Check sheet for the modelled part. Datum: model origin and axes. Units: mm. Face numbers are marked on the shaded views. A direction names the side the tool comes from. Give positions to 0.01 mm unless a question says otherwise; leave off trailing zeros. Loops run counter-clockwise (first coordinate to the right, second up) from the corner with the lowest first, then second, coordinate; pieces in that order, holes last. Notation, with made-up numbers: M 38,20 L 60,20 A23 cw 60,58 Z; hole C 23,28.5 d6. An arc over 180 degrees is marked long. Use one line per item in the form item = value.
from build123d import *

# Parameters (mm, degrees)
SKETCH_1_W             = 50
SKETCH_1_H             = 35
EXTRUDE_445_DEPTH      = 11.3
SKETCH_2_R             = 7.5
SKETCH_2_R_2           = 1.25
CUT_EXTRUDE_665_DEPTH  = 36.800698317
CUT_EXTRUDE_1135_DEPTH = 9.3
SKETCH_4_W             = 27
SKETCH_4_H             = 34.5
CUT_EXTRUDE_1595_DEPTH = 1
SKETCH_5_W             = 23
SKETCH_5_H             = 3.5
CUT_EXTRUDE_1822_DEPTH = 12.75
FILLET_1_R             = 1
FILLET_3_R             = 1
SKETCH_7_R             = 1.25
CUT_EXTRUDE_3943_DEPTH = 45.471226653
SKETCH_8_W             = 6
SKETCH_8_H             = 7.8
CUT_EXTRUDE_4259_DEPTH = 3
CHAMFER_1_SIZE         = 1
FILLET_2_R             = 2


with BuildPart() as part:
    # Эскиз1 → Extrude 445 (new body)
    with BuildSketch(Plane.XY):
        with Locations((0, 5.5)):
            Rectangle(SKETCH_1_W, SKETCH_1_H)
    extrude(amount=EXTRUDE_445_DEPTH)

    # Эскиз2 → Cut-Extrude 665 (cut, through all)
    with BuildSketch(Plane(origin=(0, 0, 0), x_dir=(-1, 0, 0), z_dir=(0, 0, -1))):
        Circle(SKETCH_2_R)
        with Locations((-10.5, 6.75)):
            Circle(SKETCH_2_R_2)
        with Locations((10.5, 6.75)):
            Circle(SKETCH_2_R_2)
        with Locations((10.5, -6.75)):
            Circle(SKETCH_2_R_2)
        with Locations((-10.5, -6.75)):
            Circle(SKETCH_2_R_2)
    extrude(amount=-CUT_EXTRUDE_665_DEPTH, mode=Mode.SUBTRACT)

    # Эскиз3 → Cut-Extrude 1135 (cut)
    with BuildSketch(Plane(origin=(0, 0, 0), x_dir=(-1, 0, 0), z_dir=(0, 0, -1))):
        with BuildLine():
            Line((-13.5, 10.25), (13.5, 10.25))
            Line((13.5, 10.25), (13.5, 8.25))
            Line((13.5, 8.25), (10.5, 8.25))
            ThreePointArc((10.5, 8.25), (9, 6.75), (10.5, 5.25))
            Line((10.5, 5.25), (13.5, 5.25))
            Line((13.5, 5.25), (13.5, -5.25))
            Line((13.5, -5.25), (10.5, -5.25))
            ThreePointArc((10.5, -5.25), (9.439339828, -5.689339828), (9, -6.75))
            Line((9, -6.75), (9, -9))
            Line((9, -9), (-9, -9))
            Line((-9, -9), (-9, -6.75))
            ThreePointArc((-9, -6.75), (-9.439339828, -5.689339828), (-10.5, -5.25))
            Line((-10.5, -5.25), (-13.5, -5.25))
            Line((-13.5, -5.25), (-13.5, 5.25))
            Line((-13.5, 5.25), (-10.5, 5.25))
            ThreePointArc((-10.5, 5.25), (-9, 6.75), (-10.5, 8.25))
            Line((-10.5, 8.25), (-13.5, 8.25))
            Line((-13.5, 8.25), (-13.5, 10.25))
        make_face()
    extrude(amount=-CUT_EXTRUDE_1135_DEPTH, mode=Mode.SUBTRACT)

    # Эскиз4 → Cut-Extrude 1595 (cut)
    with BuildSketch(Plane(origin=(0, 0, 0), x_dir=(-1, 0, 0), z_dir=(0, 0, -1))):
        with Locations((0, 5.75)):
            Rectangle(SKETCH_4_W, SKETCH_4_H)
    extrude(amount=-CUT_EXTRUDE_1595_DEPTH, mode=Mode.SUBTRACT)

    # Эскиз5 → Cut-Extrude 1822 (cut)
    with BuildSketch(Plane(origin=(0, 23, 0), x_dir=(1, 0, 0), z_dir=(0, 1, 0))):
        with Locations((0, -1.75)):
            Rectangle(SKETCH_5_W, SKETCH_5_H)
    extrude(amount=-CUT_EXTRUDE_1822_DEPTH, mode=Mode.SUBTRACT)

    # Скругление1
    fillet_1_edges = [part.edges().sort_by_distance(p)[0] for p in [
        (0, 10.25, 3.5),
        (7.5, 0, 9.3),
    ]]
    fillet(fillet_1_edges, radius=FILLET_1_R)

    # Скругление3
    fillet_3_edges = [part.edges().sort_by_distance(p)[0] for p in [
        (13.5, 9.25, 9.3),
        (13.5, 8.25, 5.15),
        (0, 10.25, 9.3),
        (-13.5, 9.25, 9.3),
        (-12, 8.25, 9.3),
        (-13.5, 8.25, 5.15),
        (-9, 6.75, 9.3),
        (-12, 5.25, 9.3),
        (-13.5, 0, 9.3),
        (-13.5, 5.25, 5.15),
        (-12, -5.25, 9.3),
        (-13.5, -5.25, 5.15),
        (-9.439339828, -5.689339828, 9.3),
        (-9, -7.875, 9.3),
        (0, -9, 9.3),
        (-9, -9, 5.15),
        (9, -7.875, 9.3),
        (9, -9, 5.15),
        (9.439339828, -5.689339828, 9.3),
        (12, -5.25, 9.3),
        (13.5, 0, 9.3),
        (13.5, -5.25, 5.15),
        (12, 5.25, 9.3),
        (13.5, 5.25, 5.15),
        (9, 6.75, 9.3),
        (12, 8.25, 9.3),
    ]]
    fillet(fillet_3_edges, radius=FILLET_3_R - 0.0001)  # a hair under: the kernel refuses the full size

    # Эскиз7 → Cut-Extrude 3943 (cut, through all)
    with BuildSketch(Plane(origin=(0, 23, 0), x_dir=(1, 0, 0), z_dir=(0, 1, 0))):
        with Locations(Location((-20, -5.65, 0), (0, 0, 180))):
            Circle(SKETCH_7_R)
        with Locations(Location((20, -5.65, 0), (0, 0, 180))):
            Circle(SKETCH_7_R)
    extrude(amount=-CUT_EXTRUDE_3943_DEPTH, mode=Mode.SUBTRACT)

    # Эскиз8 → Cut-Extrude 4259 (cut)
    with BuildSketch(Plane(origin=(0, 23, 0), x_dir=(1, 0, 0), z_dir=(0, 1, 0))):
        with Locations((0, -7.4)):
            Rectangle(SKETCH_8_W, SKETCH_8_H)
    extrude(amount=-CUT_EXTRUDE_4259_DEPTH, mode=Mode.SUBTRACT)

    # Фаска1
    chamfer_1_edges = [part.edges().sort_by_distance(p)[0] for p in [
        (11.75, 6.75, 11.3),
        (-9.25, 6.75, 11.3),
        (-9.25, -6.75, 11.3),
        (11.75, -6.75, 11.3),
    ]]
    chamfer(chamfer_1_edges, length=CHAMFER_1_SIZE)

    # Скругление2
    fillet_2_edges = [part.edges().sort_by_distance(p)[0] for p in [
        (25, 5.5, 11.3),
        (-25, 5.5, 11.3),
        (25, 5.5, 0),
        (-25, 5.5, 0),
    ]]
    fillet(fillet_2_edges, radius=FILLET_2_R)


solid = part.part
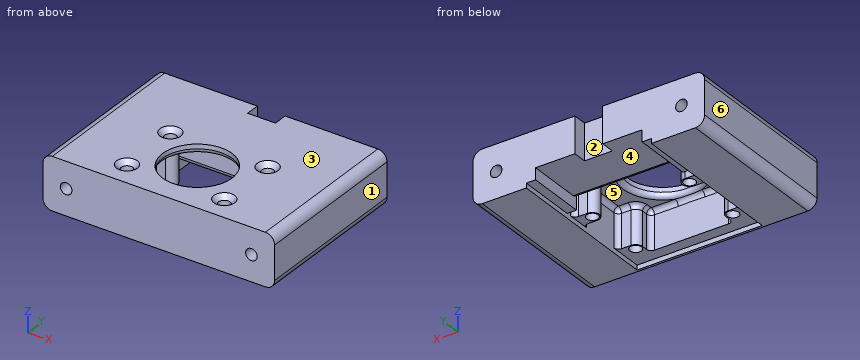
1) Scan lines: line 1 (Y direction, x = 10.5, z = 7.75); line 2 (Y direction, x = 6.5, z = 5.25). Record each from-to range of solid material in increasing order.
Evaluation:
line_1 = -12 to -8, -5.5 to -5.25, 5.25 to 5.5, 8 to 8.25, 10.25 to 23
line_2 = -12 to -9, 10.25 to 23
2) Release check for a two-part mould opening along X. For the marked faces 1, 2 and 3 record: pulls with the +X half, pulls with the -X half, needs draft (parallel to the pull), parting line crosses it, or undercut.
Evaluation:
face_1 = pulls with the +X half
face_2 = undercut
face_3 = needs draft
3) Set-up check for the marked faces 4, 5 and 6: record each of +Z, -Z, +X, -X, +Y, -Y from which the full face is reachable in a straight line by a thin tool's end or side.
Evaluation:
face_4 = -Z, +Y
face_5 = -Z
face_6 = +Z, -Z, -X, +Y, -Y
4) Depth check by flat-ended pin: pin 1 Ø13 at (x, y) = (-3, 16) entering from -Z; pin 2 Ø4 at (x, y) = (-10.5, -6.75) entering from -Z; pin 3 Ø1.5 at (x, y) = (-5.5, -4.5) entering from -Z. Enter the tip coordinate at first touch or a pass-through.
Evaluation:
pin_1 = 3.5
pin_2 = 1
pin_3 = 9.53
5) Section check B-B (x = -20). Record the cut outline in (y, z), then the cut area to 3 significant figures.
Evaluation:
outline = M -12,0 L 23,0 L 23,4.4 L -12,4.4 Z; M -12,6.9 L 23,6.9 L 23,11.3 L -12,11.3 Z
area = 308 mm^2
6) Section check D-D (y = 0). Record the cut outline in (x, z), then the cut area to 3 significant figures.
Evaluation:
outline = M -25,2 A2 ccw -23,0 L -13.5,0 L -13.5,8.3 A1 cw -12.5,9.3 L -8.5,9.3 A1 ccw -7.5,10.3 L -7.5,11.3 L -23,11.3 A2 ccw -25,9.3 Z; M 7.5,10.3 A1 ccw 8.5,9.3 L 12.5,9.3 A1 cw 13.5,8.3 L 13.5,0 L 23,0 A2 ccw 25,2 L 25,9.3 A2 ccw 23,11.3 L 7.5,11.3 Z; hole C -20,5.65 d2.5; hole C 20,5.65 d2.5
area = 271 mm^2
7) Section check C-C (y = 12.5). Record the cut outline in (x, z).
Evaluation:
outline = M -25,2 A2 ccw -23,0 L -13.5,0 L -13.5,1 L -11.5,1 L -11.5,3.5 L 11.5,3.5 L 11.5,1 L 13.5,1 L 13.5,0 L 23,0 A2 ccw 25,2 L 25,9.3 A2 ccw 23,11.3 L -23,11.3 A2 ccw -25,9.3 Z; hole C -20,5.65 d2.5; hole C 20,5.65 d2.5
8) Section check A-A (y = 20.5). Record the cut outline in (x, z).
Evaluation:
outline = M -25,2 A2 ccw -23,0 L -13.5,0 L -13.5,1 L -11.5,1 L -11.5,3.5 L -3,3.5 L -3,11.3 L -23,11.3 A2 ccw -25,9.3 Z; M 3,3.5 L 11.5,3.5 L 11.5,1 L 13.5,1 L 13.5,0 L 23,0 A2 ccw 25,2 L 25,9.3 A2 ccw 23,11.3 L 3,11.3 Z; hole C -20,5.65 d2.5; hole C 20,5.65 d2.5
